```python
from build123d import *

# Parameters (mm, degrees)
F0_R     = 8.001
F0_R_2   = 5.08
F1_DEPTH = 58.674
F2_R     = 8.001
F2_R_2   = 5.08
F3_ANGLE = -90
F4_R     = 8.001
F4_R_2   = 5.08
F5_DEPTH = 31.75


with BuildPart() as f1:
    # F0 (on Front) → F1 (new body)
    with BuildSketch(Plane.XZ):
        Circle(F0_R)
        Circle(F0_R_2, mode=Mode.SUBTRACT)
    extrude(amount=F1_DEPTH)

    # F2 (on face) → F3 (revolve)
    with BuildSketch(Plane.XZ.offset(58.674)):
        Circle(F2_R)
        Circle(F2_R_2, mode=Mode.SUBTRACT)
    revolve(axis=Axis((19.05, -58.674, -0.586418), (0, 0, -1)), revolution_arc=F3_ANGLE)

    # F4 (on face) → F5 (join)
    with BuildSketch(Plane.YZ.offset(19.05)):
        with Locations((-77.724, 0)):
            Circle(F4_R)
        with Locations((-77.724, 0)):
            Circle(F4_R_2, mode=Mode.SUBTRACT)
    extrude(amount=F5_DEPTH)


solid = f1.part
```
The listing builds one solid part. Answer for the finished solid, in the listing's coordinates (mm). A direction names the side the tool comes from. Round coordinates to 2 decimals unless told otherwise and drop trailing zeros. Loops run counter-clockwise (first coordinate to the right, second up) from the corner with the lowest first, then second, coordinate; pieces in that order, holes last.
Q1. Given pin 1 Ø1.5 at (y, z) = (-15, -4.5) entering from -X; pin 2 Ø1.5 at (x, y) = (10, -76.5) entering from +Z; pin 3 Ø6 at (y, z) = (-27.5, -4) entering from -X; pin 4 Ø4 at (y, z) = (-35.5, -1) entering from -X, each flat-ended and moving along its own axis, determine where each tip first touches the part or whether it passes through.
Q2. Section D-D, the plane z = 6.25 is taken. Determine the outline of the cut face in (x, y), then the cut area to 3 significant figures.
Q3. Section C-C, the plane z = 0 is taken. Determine the outline of the cut face in (x, y) (3 decimals).
Q4. For a pull along X with two mould halves and no side action, classify faces 1 (the face through (34.7, -82.8, 0.2)), 2 (the face through (-0.661, -28.926, 5.037)), 3 (the face through (-1.73, -28.93, -7.81)) as released by +X, released by -X, zero draft, split by the parting line, or undercut.
Q5. Section B-B, the plane y = -17.5 is taken. Determine the outline of the cut face in (x, z).
Q6. Find the intervals of material crossed by line 1 (Z direction, x = 0, y = -34); line 2 (Z direction, x = -3, y = -39); line 3 (X direction, y = -41.5, z = 1.25), in increasing order.
Q7. Which of the six approach directions +Z, -Z, +X, -X, +Y, -Y give full straight-line access (tool end or side, diameter ignored) to faces 4 (the face through (34.703, -85.717, 0.352)), 5 (the face through (50.8, -76, -5))?
Q8. Section A-A, the plane z = -4 is taken. Determine the outline of the cut face in (x, y), then the cut area to 3 significant figures.
Completed:
1. pin 1: stops at x = -7.07
1. pin 2: stops at z = 8
1. pin 3: stops at x = -7.94
1. pin 4: stops at x = -8
2. outline: (-5, -58.67) arc R24.05 ccw to (19.05, -82.72) - (50.8, -82.72) - (50.8, -72.73) - (19.05, -72.73) arc R14.05 cw to (5, -58.67) - (5, 0) - (-5, 0) - close
2. area: 1,200 mm2
3. outline: (-8.001, -58.674) arc R27.051 ccw to (19.05, -85.725) - (50.8, -85.725) - (50.8, -82.804) - (19.05, -82.804) arc R24.13 cw to (-5.08, -58.674) - (-5.08, 0) - (-8.001, 0) - close; (5.08, -58.674) arc R13.97 ccw to (19.05, -72.644) - (50.8, -72.644) - (50.8, -69.723) - (19.05, -69.723) arc R11.049 cw to (8.001, -58.674) - (8.001, 0) - (5.08, 0) - close
4. face 1: zero draft
4. face 2: undercut
4. face 3: split by the parting line
5. outline: circle Ø16 at (0, 0); hole circle Ø10.16 at (0, 0)
6. line 1: z = -8 to -5.08, 5.08 to 8
6. line 2: z = -7.42 to -4.1, 4.1 to 7.42
6. line 3: x = -7.9 to -4.92, 4.92 to 7.9
7. face 4: +X
7. face 5: +Z, -Z, +X, +Y, -Y
8. outline: (-6.93, -58.67) arc R25.98 ccw to (19.05, -84.65) - (50.8, -84.65) - (50.8, -80.86) - (19.05, -80.86) arc R22.18 cw to (-3.13, -58.67) - (-3.13, 0) - (-6.93, 0) - close; (3.13, -58.67) arc R15.92 ccw to (19.05, -74.59) - (50.8, -74.59) - (50.8, -70.79) - (19.05, -70.79) arc R12.12 cw to (6.93, -58.67) - (6.93, 0) - (3.13, 0) - close
8. area: 914 mm2
